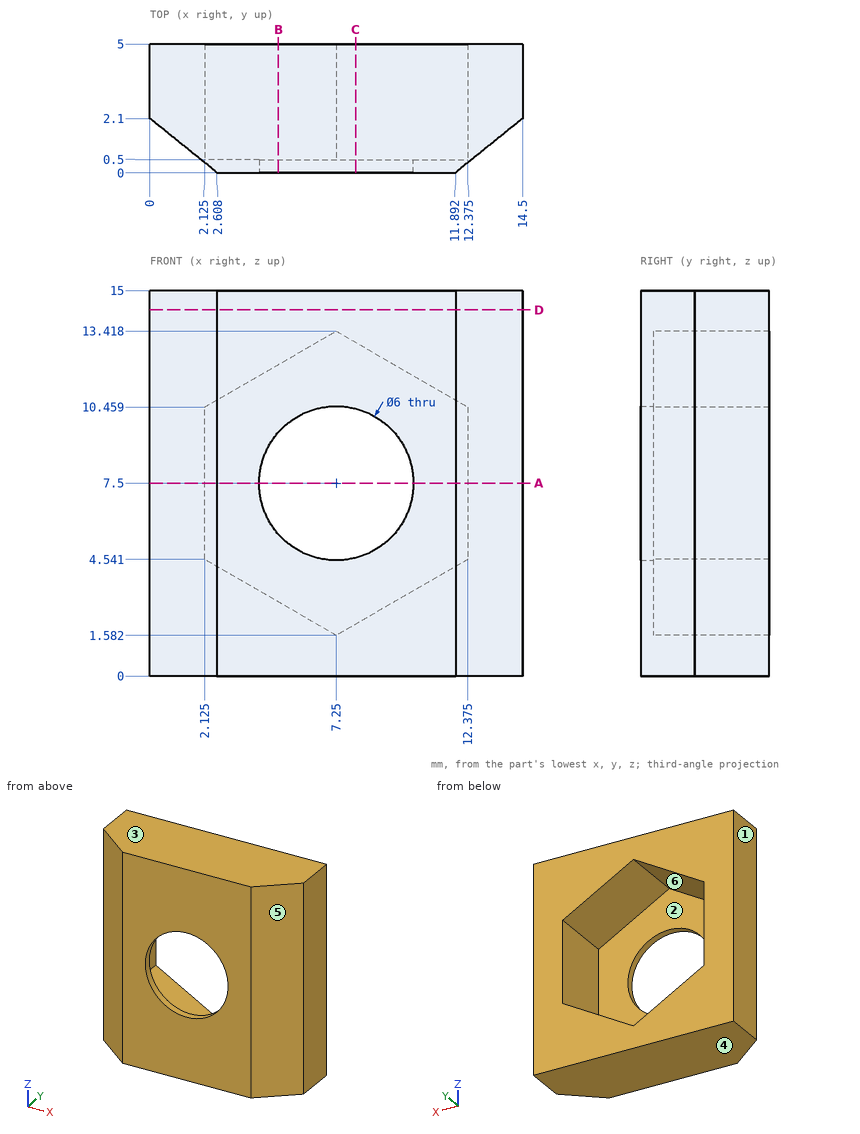
Geometry check sheet. Reference: drawing and pictorial views, mm from the part's lowest x, y, z. A direction names the side the tool comes from. Give positions to 0.01 mm unless a question says otherwise; leave off trailing zeros. Write each loop counter-clockwise with the first axis right and the second up, starting at its lowest first coordinate (ties: lowest second). Pieces come first, ordered by that corner, then holes.
Item 1: Access from +Z, -Z, +X, -X, +Y, -Y to the whole of each face (thin tool, end or side, straight path). Record for the marked faces 1 and 2.
Item 2: Scan lines: L1, parallel to Z at x = 7.25, y = 0.25; L2, parallel to X at y = 3.3, z = 5 (3 decimals); L3, parallel to X at y = 3.15, z = 2.5. Record each from-to range of solid material in increasing order.
Item 3: Draft check along Z on the marked faces 3, 4, 5 and 6. Enter one of: released by +Z, released by -Z, zero draft, split by the parting line, or undercut.
Item 4: Cross-section at D-D (z = 14.25). Enter the section's corners in (x, y).
Item 5: Cross-section at B-B (x = 5). Enter the section's corners in (y, z).
Item 6: Cross-section at A-A (z = 7.5). Enter the section's corners in (x, y) (3 decimals), and give its area (3 significant figures).
Item 7: Gauge pin test, flat ends, axial feed: pin 1 (2 mm diameter, centred on y = 1, z = 8.5, fed in from +X); pin 2 (7 mm diameter, centred on x = 7.25, z = 7.5, fed in from +Y). Record the tip position at first contact, or that the pin passes through.
Item 8: Cross-section at C-C (x = 8). Enter the section's corners in (y, z) (1 decimal), and give its area (3 significant figures).
Report:
1. face 1: +Z, -Z, -X, +Y, -Y
1. face 2: +Y
2. L1: z = 0 to 4.5, 10.5 to 15
2. L2: x = 0 to 2.125, 12.375 to 14.5
2. L3: x = 0 to 5.66, 8.84 to 14.5
3. face 3: released by +Z
3. face 4: released by -Z
3. face 5: zero draft
3. face 6: undercut
4. outline: (0, 2.1) - (2.61, 0) - (11.89, 0) - (14.5, 2.1) - (14.5, 5) - (0, 5) - close
5. outline: (0, 0) - (5, 0) - (5, 2.88) - (0.5, 2.88) - (0.5, 5.52) - (0, 5.52) - close; (0, 9.48) - (0.5, 9.48) - (0.5, 12.12) - (5, 12.12) - (5, 15) - (0, 15) - close
6. outline: (0, 2.1) - (2.608, 0) - (4.25, 0) - (4.25, 0.5) - (2.125, 0.5) - (2.125, 5) - (0, 5) - close; (10.25, 0) - (11.892, 0) - (14.5, 2.1) - (14.5, 5) - (12.375, 5) - (12.375, 0.5) - (10.25, 0.5) - close
6. area: 17.9 mm2
7. pin 1: stops at x = 14.38
7. pin 2: stops at y = 0.5
8. outline: (0, 0) - (5, 0) - (5, 2) - (0.5, 2) - (0.5, 4.6) - (0, 4.6) - close; (0, 10.4) - (0.5, 10.4) - (0.5, 13) - (5, 13) - (5, 15) - (0, 15) - close
8. area: 22.7 mm2
